The figure shows three views and two pictorial views of one solid part (mm, origin at its lowest corner). Answer the questions. Round coordinates to 2 decimals unless told otherwise and drop trailing zeros. Order: outer loops, then holes, each group sorted by start corner. A loop starts at its lowest first (then second) coordinate and runs counter-clockwise, first axis right, second up. Notation, with made-up numbers: (-1, 17.5) -> (22, 17.5) arc R10 cw to (22, 21.5) -> close; hole circle Ø6 at (57, -39.75). An arc over 180 degrees is marked (long way). Return JSON: item names as keys, results as strings. Group by question number.
(1) The part is cut by section A-A (z = 43). Determine the outline of the cut face in (x, y).
(2) Consider line 1 (Z direction, x = 43, y = 1.6); line 2 (X direction, y = 1.2, z = 93.5); line 3 (X direction, y = 0.55, z = 46). Determine where each line is inside the solid, lowest interval first. Write a range as [from, to].
(3) Each of these flat-tipped pins is pushed along its axis until it touches: pin 1 (1.5 mm diameter, centred on x = 84.5, y = 2, fed in from +Z); pin 2 (1.5 mm diameter, centred on x = 2, y = 2, fed in from -Z); pin 3 (1.5 mm diameter, centred on y = 2, z = 98.5, fed in from +X). Where does it stop, or does it pass through?
(4) The part is cut by section B-B (x = 43). Determine the outline of the cut face in (y, z), plus the area to 3 significant figures.
(5) The part is cut by section C-C (x = 78.5). Determine the outline of the cut face in (y, z), plus the area to 3 significant figures.
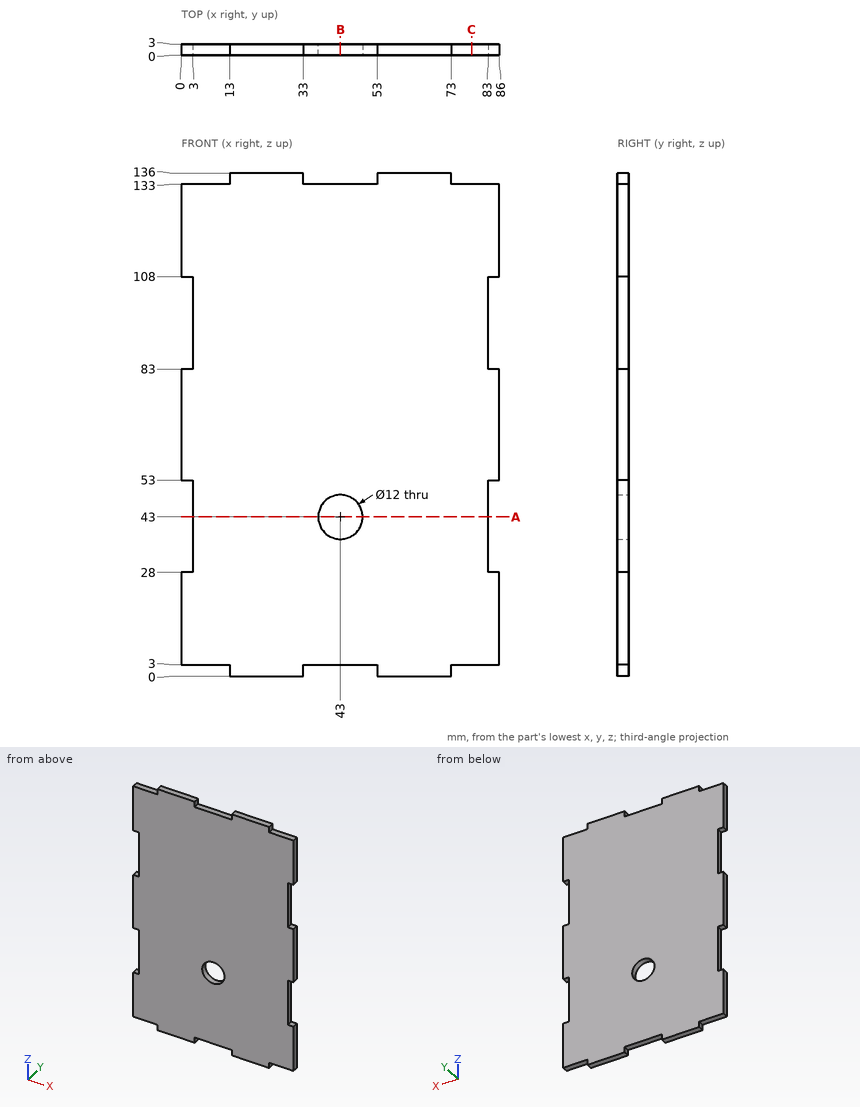
Answer below:
{
 "1": {"outline": "(3, 0) -> (37, 0) -> (37, 3) -> (3, 3) -> close; (49, 0) -> (83, 0) -> (83, 3) -> (49, 3) -> close"},
 "2": {"line 1": "z = [3, 37], [49, 133]", "line 2": "x = [3, 83]", "line 3": "x = [3, 37.8], [48.2, 83]"},
 "3": {"pin 1": "stops at z = 133", "pin 2": "stops at z = 3", "pin 3": "stops at x = 83"},
 "4": {"outline": "(0, 3) -> (3, 3) -> (3, 37) -> (0, 37) -> close; (0, 49) -> (3, 49) -> (3, 133) -> (0, 133) -> close", "area": "354 mm²"},
 "5": {"outline": "(0, 3) -> (3, 3) -> (3, 133) -> (0, 133) -> close", "area": "390 mm²"}
}
